```python
from build123d import *

# Parameters (mm, degrees)
F1_DEPTH = 100
F2_R     = 3.5
F3_DEPTH = 30.001
F4_R     = 8
F5_DEPTH = 50.001
F7_DEPTH = 3
F9_DEPTH = 3


with BuildPart() as f1:
    # F0 (on Right) → F1 (new body)
    with BuildSketch(Plane.YZ):
        Polygon((0, 0), (-50, 0), (-50, -5), (-5, -5), (-5, -30), (0, -30), align=None)
    extrude(amount=F1_DEPTH)

    # F2 (on face) → F3 (cut, through all)
    with BuildSketch(Plane.XY):
        with Locations((10, -35)):
            Circle(F2_R)
        with Locations((10, -15)):
            Circle(F2_R)
        with Locations((90, -35)):
            Circle(F2_R)
        with Locations((90, -15)):
            Circle(F2_R)
    extrude(amount=-F3_DEPTH, mode=Mode.SUBTRACT)

    # F4 (on face) → F5 (cut, through all)
    with BuildSketch(Plane(origin=(0, 0, 0), x_dir=(-1, 0, 0), z_dir=(0, 1, 0))):
        with Locations((-50, -15)):
            Circle(F4_R)
    extrude(amount=-F5_DEPTH, mode=Mode.SUBTRACT)

    # F6 (on face) → F7 (join)
    with BuildSketch(Plane.YZ.offset(100)):
        Polygon((0, 0), (-50, 0), (-50, -5), (-5, -30), (0, -30), align=None)
    extrude(amount=F7_DEPTH)

    # F8 (on face) → F9 (join)
    with BuildSketch(Plane(origin=(0, 0, 0), x_dir=(0, -1, 0), z_dir=(-1, 0, 0))):
        Polygon((50, -5), (50, 0), (0, 0), (0, -30), (5, -30), align=None)
    extrude(amount=F9_DEPTH)


solid = f1.part
```
Source: CAD feature listing. Evaluate the final solid. Frame: model axes, mm. A direction names the side the tool comes from. Round coordinates to 2 decimals unless told otherwise and drop trailing zeros. Write each loop counter-clockwise with the first axis right and the second up, starting at its lowest first coordinate (ties: lowest second). Pieces come first, ordered by that corner, then holes. Notation, with made-up numbers: M -28,59 L -3,59 A21 ccw -3,91 Z; hole C -36.5,59.25 d9. An arc over 180 degrees is marked long. Answer as a JSON object with one key per item and string values. Group by question number.
(1) Section query C-C on y = -35. Output: boundary loops of the cut face in (x, z).
(2) Reachability of faces 1 (the flat face through (100, -18, -12)), 2 (the cylindrical face through (56.349, -2.465, -19.868)) from +Z, -Z, +X, -X, +Y, -Y: full face, straight path, thin tool, end or side. Return the list, or none.
(3) Mould query, pull axis X, two halves, no side actions, for faces 3 (the flat face through (51, -25, 0)), 4 (the flat face through (103, -20, -11)), 5 (the flat face through (49, -5, -26)). Classes: +X half, -X half, draft (parallel to the pull), parting line (faces both ways), or undercut.
(4) Section query B-B on z = -3.5. Output: boundary loops of the cut face in (x, y), then the cut area to 3 significant figures.
(5) Section query D-D on z = -15. Output: boundary loops of the cut face in (x, y), then the cut area to 3 significant figures.
(6) First-contact query: pin 1 (9 mm diameter, centred on x = 90, y = -35, fed in from -Z); pin 2 (7.5 mm diameter, centred on x = 64, z = -18, fed in from -Y). Flat tips, straight axial feed; report the tip coordinate or a pass-through.
(7) Section query A-A on x = 90. Output: boundary loops of the cut face in (y, z), then the cut area to 3 significant figures.
(8) Ray query, line 1 (Y direction, x = 10, z = -3.35); line 2 (X direction, y = -15.5, z = -3.5); line 3 (Z direction, x = 72, y = -38). Return the intervals inside material, ascending. Write a range as [from, to].
Computed values:
{
 "1": {"outline": "M -3,-13.33 L 0,-13.33 L 0,-5 L 6.5,-5 L 6.5,0 L -3,0 Z; M 13.5,-5 L 86.5,-5 L 86.5,0 L 13.5,0 Z; M 93.5,-5 L 100,-5 L 100,-13.33 L 103,-13.33 L 103,0 L 93.5,0 Z"},
 "2": {"face 1": "-Z, -Y", "face 2": "+Y, -Y"},
 "3": {"face 3": "draft", "face 4": "+X half", "face 5": "undercut"},
 "4": {"outline": "M -3,-50 L 103,-50 L 103,0 L -3,0 Z; hole C 10,-35 d7; hole C 10,-15 d7; hole C 90,-35 d7; hole C 90,-15 d7", "area": "5,150 mm^2"},
 "5": {"outline": "M -3,-32 L 0,-32 L 0,-5 L 42,-5 L 42,0 L -3,0 Z; M 58,-5 L 100,-5 L 100,-32 L 103,-32 L 103,0 L 58,0 Z", "area": "612 mm^2"},
 "6": {"pin 1": "z = -5", "pin 2": "y = -5"},
 "7": {"outline": "M -50,-5 L -38.5,-5 L -38.5,0 L -50,0 Z; M -31.5,-5 L -18.5,-5 L -18.5,0 L -31.5,0 Z; M -11.5,-5 L -5,-5 L -5,-30 L 0,-30 L 0,0 L -11.5,0 Z", "area": "305 mm^2"},
 "8": {"line 1": "[-50, -38.5], [-31.5, -18.5], [-11.5, 0]", "line 2": "[-3, 6.54], [13.46, 86.54], [93.46, 103]", "line 3": "[-5, 0]"}
}
